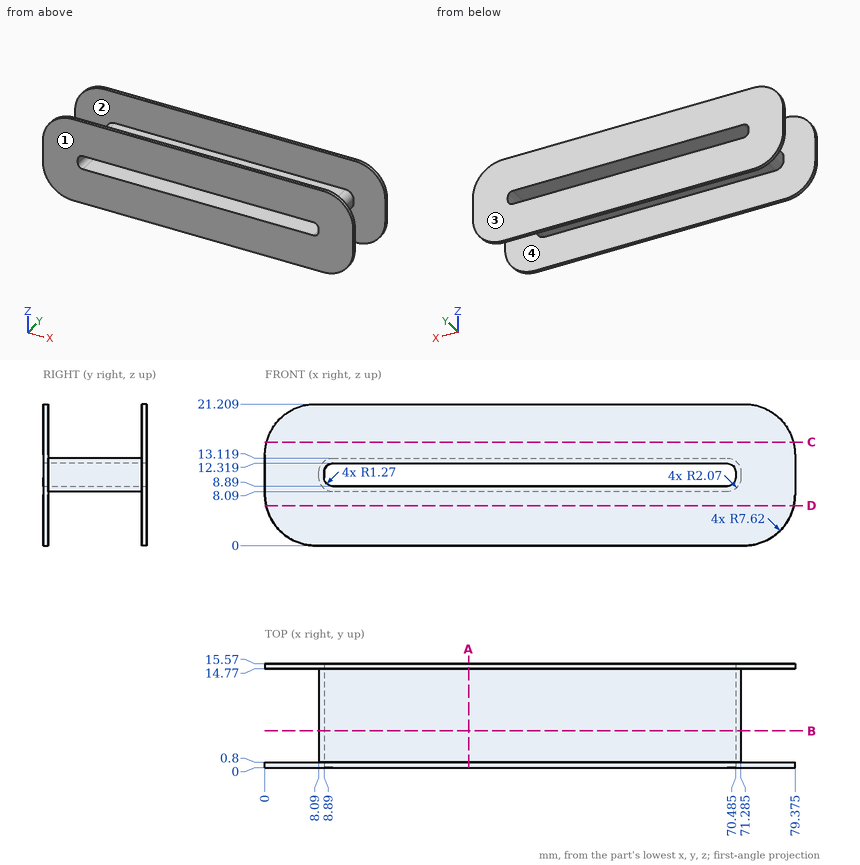
The drawing under review shows one solid part. Ordinate dimensions are in mm from its lowest x, y, z. Give positions to 0.01 mm unless a question says otherwise; leave off trailing zeros. Loops run counter-clockwise (first coordinate to the right, second up) from the corner with the lowest first, then second, coordinate; pieces in that order, holes last. Notation, with made-up numbers: M -20.75,-28 L 16.25,-28 A21 ccw 16.25,-2 Z; hole C 36,43 d6. An arc over 180 degrees is marked long. Return JSON: item names as keys, results as strings. Group by question number.
Item 1: We need section A-A (x = 30.5). Give the boundary of the cut face in (y, z).
Item 2: Insertion check: pin 1 Ø2 at (x, z) = (42, 7) entering from -Y; pin 2 Ø1.5 at (x, y) = (57, 9.5) entering from +Z; pin 3 Ø4 at (x, y) = (32.5, 7) entering from -Z; pin 4 Ø0.7 at (y, z) = (7.5, 10.5) entering from +X (3 decimals). Each pin has a flat end and moves straight along its axis. Give the tip position at first contact, or say it passes through.
Item 3: Mouldability with a two-part tool opening along Y and no side actions: class the marked faces 1, 2, 3 and 4 as released by +Y, released by -Y, zero draft, split by the parting line, or undercut.
Item 4: We need section D-D (z = 6). Give the boundary of the cut face in (x, y).
Item 5: For probe 1 along Z at (x, y) = (64, 11.5); probe 2 along Y at (x, z) = (36.5, 3); probe 3 along X at (y, z) = (14, 11.25), list the stretches that pass through material, from the lowest coordinate up.
Item 6: We need section C-C (z = 15.5). Give the boundary of the cut face in (x, y), and give its area (3 significant figures).
Item 7: We need section B-B (y = 5.5). Give the boundary of the cut face in (x, z) (3 decimals).
Output:
{
 "1": {"outline": "M 0,0 L 0.8,0 L 0.8,8.09 L 14.77,8.09 L 14.77,0 L 15.57,0 L 15.57,8.89 L 0,8.89 Z; M 0,12.32 L 15.57,12.32 L 15.57,21.21 L 14.77,21.21 L 14.77,13.12 L 0.8,13.12 L 0.8,21.21 L 0,21.21 Z"},
 "2": {"pin 1": "stops at y = 0", "pin 2": "stops at z = 13.12", "pin 3": "stops at z = 8.09", "pin 4": "stops at x = 71.285"},
 "3": {"face 1": "released by -Y", "face 2": "undercut", "face 3": "released by +Y", "face 4": "undercut"},
 "4": {"outline": "M 0.17,0 L 79.2,0 L 79.2,0.8 L 0.17,0.8 Z; M 0.17,14.77 L 79.2,14.77 L 79.2,15.57 L 0.17,15.57 Z"},
 "5": {"probe 1": "z = 8.09 to 8.89, 12.32 to 13.12", "probe 2": "y = 0 to 0.8, 14.77 to 15.57", "probe 3": "x = 8.1 to 8.91, 70.47 to 71.28"},
 "6": {"outline": "M 0.24,0 L 79.13,0 L 79.13,0.8 L 0.24,0.8 Z; M 0.24,14.77 L 79.13,14.77 L 79.13,15.57 L 0.24,15.57 Z", "area": "126 mm^2"},
 "7": {"outline": "M 8.09,10.16 A2.07 ccw 10.16,8.09 L 69.215,8.09 A2.07 ccw 71.285,10.16 L 71.285,11.049 A2.07 ccw 69.215,13.119 L 10.16,13.119 A2.07 ccw 8.09,11.049 Z; hole M 8.89,10.16 A1.27 ccw 10.16,8.89 L 69.215,8.89 A1.27 ccw 70.485,10.16 L 70.485,11.049 A1.27 ccw 69.215,12.319 L 10.16,12.319 A1.27 ccw 8.89,11.049 Z"}
}
